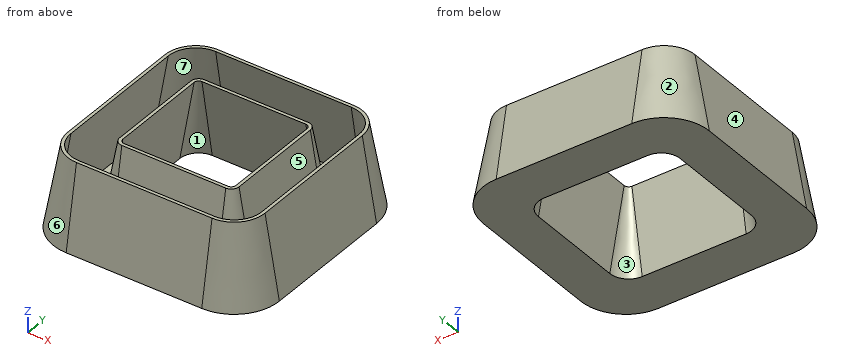
from build123d import *

# Parameters (mm, degrees)
F1_DEPTH = 18
F1_TAPER = 10
F3_DEPTH = 18.001
F3_TAPER = -10
F4_T     = -0.7


with BuildPart() as f1:
    # F0 (on Top) → F1 (new body)
    with BuildSketch(Plane.XY):
        with BuildLine():
            ThreePointArc((25, 15), (22.0710678119, 22.0710678119), (15, 25))
            Line((15, 25), (-15, 25))
            ThreePointArc((-15, 25), (-22.0710678119, 22.0710678119), (-25, 15))
            Line((-25, 15), (-25, -15))
            ThreePointArc((-25, -15), (-22.0710678119, -22.0710678119), (-15, -25))
            Line((-15, -25), (15, -25))
            ThreePointArc((15, -25), (22.0710678119, -22.0710678119), (25, -15))
            Line((25, -15), (25, 15))
        make_face()
    extrude(amount=F1_DEPTH, taper=F1_TAPER)

    # F2 (on face) → F3 (cut, through all)
    with BuildSketch(Plane.XY.offset(18)):
        with BuildLine():
            ThreePointArc((12.5, 11), (12.2071067812, 11.7071067812), (11.5, 12))
            Line((11.5, 12), (-11.5, 12))
            ThreePointArc((-11.5, 12), (-12.2071067812, 11.7071067812), (-12.5, 11))
            Line((-12.5, 11), (-12.5, -11))
            ThreePointArc((-12.5, -11), (-12.2071067812, -11.7071067812), (-11.5, -12))
            Line((-11.5, -12), (11.5, -12))
            ThreePointArc((11.5, -12), (12.2071067812, -11.7071067812), (12.5, -11))
            Line((12.5, -11), (12.5, 11))
        make_face()
    extrude(amount=-F3_DEPTH, taper=F3_TAPER, mode=Mode.SUBTRACT)

    # F4
    f4_openings = [f1.faces().sort_by_distance(p)[0] for p in [
        (21.208779, 0, 18),
    ]]
    offset(amount=F4_T, openings=f4_openings)


solid = f1.part
Model file for the job. Use its own axes, mm. Face numbers are marked on the shaded views. A direction names the side the tool comes from. Round coordinates to 2 decimals unless told otherwise and drop trailing zeros. Write each question's results on one line, items separated by ' | '.
(1) Mould opens along Y. For the marked faces 1, 2, 3 and 4 say: released by +Y, released by -Y, zero draft, split by the parting line, or undercut.
Answer below:
face 1: undercut | face 2: released by +Y | face 3: undercut | face 4: zero draft
(2) Saw through at A-A, the plane z = 13.5. Count the separate pieces of the cut face and the enclosed holes in it, then the cut area to 3 significant figures.
Answer below:
separate pieces: 2 | enclosed holes: 2 | area: 191 mm^2
(3) Pin check, flat tips, straight feed: pin 1 (1 mm diameter, centred on y = 0, z = 13, fed in from -X); pin 2 (1 mm diameter, centred on x = -0.5, z = 13.5, fed in from -Y); pin 3 (5 mm diameter, centred on x = -19, z = 2.5, fed in from +Y). Stop position of each tip, or through.
Answer below:
pin 1: stops at x = -22.8 | pin 2: stops at y = -22.71 | pin 3: stops at y = 24.62
(4) 3-axis set-ups, long thin cutter, end or side, ignore diameter. For the marked faces 5, 6 and 7: which of +Z, -Z, +X, -X, +Y, -Y reach the whole face in a straight line?
Answer below:
face 5: +Z | face 6: +Z, -X, -Y | face 7: none
(5) Wall check: L1, parallel to X at y = 13.5, z = 5; L2, parallel to Y at x = -4, z = 5.75; L3, parallel to Y at x = -4, z = 7. Give the ranges that are in metal, low to high.
Answer below:
L1: x = -24.12 to -23.41, -14.63 to -13.64, 13.64 to 14.63, 23.41 to 24.12 | L2: y = -23.99 to -23.28, -14.87 to -14.16, 14.16 to 14.87, 23.28 to 23.99 | L3: y = -23.77 to -23.05, -14.65 to -13.94, 13.94 to 14.65, 23.05 to 23.77
